Verification items for this drawing (mm, ordinates from the low corner). Give positions to 0.01 mm unless a question says otherwise; leave off trailing zeros. Write each loop counter-clockwise with the first axis right and the second up, starting at its lowest first coordinate (ties: lowest second). Pieces come first, ordered by that corner, then holes. Notation, with made-up numbers: (-25.5, 72.25) -> (20.5, 72.25) arc R16 cw to (20.5, 90.25) -> close; hole circle Ø11 at (69.25, 53.5). An arc over 180 degrees is marked (long way). Write item = value, one per line.
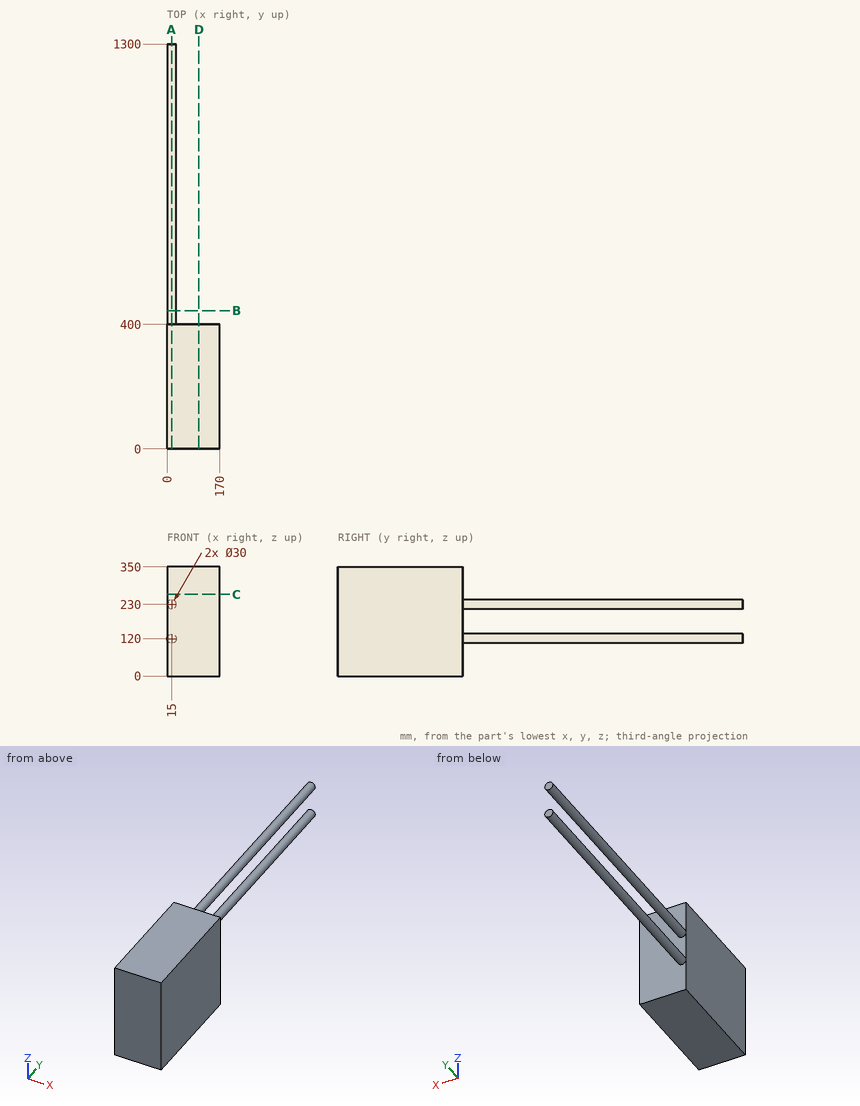
Item 1: Sectioned sample at C-C on z = 262. Record the cut outline in (x, y), then the cut area to 3 significant figures.
Response values:
outline = (0, 0) -> (170, 0) -> (170, 400) -> (0, 400) -> close
area = 68,000 mm^2
Item 2: Go/stop test with flat-tipped pins: P1, Ø1, axis at x = 128.5, z = 143, coming from the +Y side; P2, Ø3, axis at x = 90, z = 84, coming from the -Y side. Record where each tip stops, or that it passes through.
Response values:
P1 = 400
P2 = 0
Item 3: Sectioned sample at D-D on x = 102. Record the cut outline in (y, z).
Response values:
outline = (0, 0) -> (400, 0) -> (400, 350) -> (0, 350) -> close
Item 4: Sectioned sample at A-A on x = 15. Record the cut outline in (y, z), then the cut area to 3 significant figures.
Response values:
outline = (0, 0) -> (400, 0) -> (400, 105) -> (1300, 105) -> (1300, 135) -> (400, 135) -> (400, 215) -> (1300, 215) -> (1300, 245) -> (400, 245) -> (400, 350) -> (0, 350) -> close
area = 194,000 mm^2
Item 5: Material ranges on line 1 (Z direction, x = 16, y = 1198); line 2 (Y direction, x = 50, z = 161.5); line 3 (Z direction, x = 28, y = 568), recorded low to high.
Response values:
line_1 = 105.03 to 134.97, 215.03 to 244.97
line_2 = 0 to 400
line_3 = 112.52 to 127.48, 222.52 to 237.48
Item 6: Sectioned sample at B-B on y = 444. Record the cut outline in (x, z), then the cut area to 3 significant figures.
Response values:
outline = circle Ø30 at (15, 120); circle Ø30 at (15, 230)
area = 1,410 mm^2
